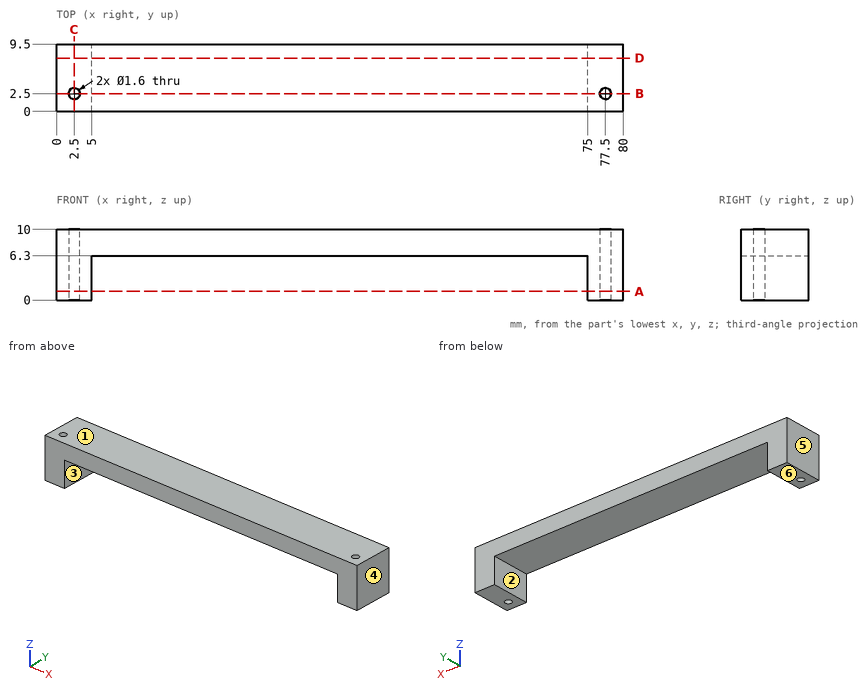
Print and shaded views of the part. All mm, measured from the part's lowest x, y and z. A direction names the side the tool comes from. Give positions to 0.01 mm unless a question says otherwise; leave off trailing zeros. Loops run counter-clockwise (first coordinate to the right, second up) from the corner with the lowest first, then second, coordinate; pieces in that order, holes last. Notation, with made-up numbers: (7.25, -37) - (11.25, -37) arc R18 cw to (11.25, -8) - close; hole circle Ø1 at (-8, 53.25). An arc over 180 degrees is marked (long way). One line per item, written item: value. Start each with the question number.
1. Slice it at C-C (x = 2.5). List the corners of the cut face in (y, z), plus the area to 3 significant figures.
2. Slice it at B-B (y = 2.5). List the corners of the cut face in (x, z).
3. Slice it at D-D (y = 7.5). List the corners of the cut face in (x, z).
4. Probe L1, parallel to X at y = 2.5, z = 2.75; L2, parallel to Y at x = 2.5, z = 4.5; L3, parallel to X at y = 4, z = 4. List the from-to ranges inside material, lowest first. Write a range as from..to.
5. Which spindle directions (+Z, -Z, +X, -X, +Y, -Y) get a long thin tool onto all of the face, cutting with end or side? Do the marked faces 1 and 2. Say none if no direction does.
6. Pull direction X, two halves, no side cores. Call the marked faces 3, 4, 5 and 6: pulls with the +X half, pulls with the -X half, needs draft (parallel to the pull), parting line crosses it, or undercut.
7. Slice it at A-A (z = 1.25). List the corners of the cut face in (x, y), plus the area to 3 significant figures.
8. Pin check, flat tip, straight feed: pin 1 (2 mm diameter, centred on x = 8.5, y = 2, fed in from -Z). Stop position of the tip, or through.
Solution:
1. outline: (0, 0) - (1.7, 0) - (1.7, 10) - (0, 10) - close; (3.3, 0) - (9.5, 0) - (9.5, 10) - (3.3, 10) - close
1. area: 79.0 mm^2
2. outline: (0, 0) - (1.7, 0) - (1.7, 10) - (0, 10) - close; (3.3, 0) - (5, 0) - (5, 6.3) - (75, 6.3) - (75, 0) - (76.7, 0) - (76.7, 10) - (3.3, 10) - close; (78.3, 0) - (80, 0) - (80, 10) - (78.3, 10) - close
3. outline: (0, 0) - (5, 0) - (5, 6.3) - (75, 6.3) - (75, 0) - (80, 0) - (80, 10) - (0, 10) - close
4. L1: x = 0..1.7, 3.3..5, 75..76.7, 78.3..80
4. L2: y = 0..1.7, 3.3..9.5
4. L3: x = 0..5, 75..80
5. face 1: +Z, +X, -X, +Y, -Y
5. face 2: -Z, +Y, -Y
6. face 3: undercut
6. face 4: pulls with the +X half
6. face 5: pulls with the -X half
6. face 6: needs draft
7. outline: (0, 0) - (5, 0) - (5, 9.5) - (0, 9.5) - close; (75, 0) - (80, 0) - (80, 9.5) - (75, 9.5) - close; hole circle Ø1.6 at (2.5, 2.5); hole circle Ø1.6 at (77.5, 2.5)
7. area: 91.0 mm^2
8. pin 1: stops at z = 6.3
